The model under review builds one solid part; all positions refer to its coordinate system, in mm. Face numbers are marked on the shaded views. A direction names the side the tool comes from. Round coordinates to 2 decimals unless told otherwise and drop trailing zeros. Write each loop counter-clockwise with the first axis right and the second up, starting at its lowest first coordinate (ties: lowest second). Pieces come first, ordered by that corner, then holes. Notation, with made-up numbers: M 67.5,73.5 L 99.5,73.5 A24 cw 99.5,101.5 Z; hole C 78,46 d7. An arc over 180 degrees is marked long. One line per item, written item: value. Start each with the question number.
1) Tool access review of the marked faces 1 and 2: name each direction out of +Z, -Z, +X, -X, +Y, -Y from which nothing blocks a thin tool from reaching the whole face with its end or side.
2) Take a section at A-A, the plane x = 0. Write out the cut boundary in (y, z), and give its area (3 significant figures).
3) Wall thickness on probe 1 along Y at (x, z) = (1.9, 1.25); probe 2 along Z at (x, y) = (-0.1, 5.75); probe 3 along Z at (x, y) = (0.65, 10.25): over which ranges is each line inside the solid? List them lowest first.
4) Take a section at B-B, the plane z = 0. Write out the cut boundary in (x, y), and give its area (3 significant figures).
5) Take a section at C-C, the plane y = 1.75. Write out the cut boundary in (x, z), and give its area (3 significant figures).
6) For P1, Ø1.5, axis at x = 1.5, y = 6.5, coming from the +Z side; P2, Ø1, axis at y = 5, z = -1.5, coming from the +X side, all flat-tipped, find the tip position at first contact; note any pin that passes through.
from build123d import *

# Parameters (mm, degrees)
SKETCH_1_W      = 2.75
SKETCH_1_H      = 1.5
SKETCH_2_R      = 1.5
EXTRUDE_1_DEPTH = 10
FILLET_1_R      = 0.367346939


with BuildPart() as part:
    # 草图1 → 旋转1 (revolve)
    with BuildSketch(Plane.XY):
        with Locations((1.375, 0.75)):
            Rectangle(SKETCH_1_W, SKETCH_1_H)
    revolve(axis=Axis((0, 1.5, 0), (0, -1, 0)))

    # 草图2 → 凸台-拉伸1 (add)
    with BuildSketch(Plane(origin=(0, 1.5, 0), x_dir=(-1, 0, 0), z_dir=(0, 1, 0))):
        Circle(SKETCH_2_R)
    extrude(amount=EXTRUDE_1_DEPTH)

    # 圆角1
    fillet_1_edges = [part.edges().sort_by_distance(p)[0] for p in [
        (-2.75, 0, 0),
    ]]
    fillet(fillet_1_edges, radius=FILLET_1_R)


solid = part.part
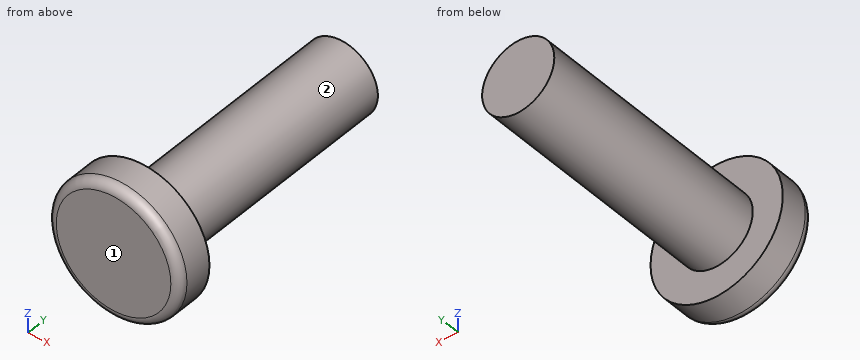
Checked values:
1. face 1: +Z, -Z, +X, -X, -Y
1. face 2: +Y
2. outline: M 0,-2.38 A0.37 ccw 0.37,-2.75 L 1.5,-2.75 L 1.5,-1.5 L 11.5,-1.5 L 11.5,1.5 L 1.5,1.5 L 1.5,2.75 L 0.37,2.75 A0.37 ccw 0,2.38 Z
2. area: 38.2 mm2
3. probe 1: y = 0 to 1.5
3. probe 2: z = -1.5 to 1.5
3. probe 3: z = -1.35 to 1.35
4. outline: M -2.75,0.37 A0.37 ccw -2.38,0 L 2.38,0 A0.37 ccw 2.75,0.37 L 2.75,1.5 L 1.5,1.5 L 1.5,11.5 L -1.5,11.5 L -1.5,1.5 L -2.75,1.5 Z
4. area: 38.2 mm2
5. outline: C 0,0 d3
5. area: 7.07 mm2
6. P1: stops at z = 1.3
6. P2: stops at x = 1.12
